The model under review builds one solid part; all positions refer to its coordinate system, in mm. Face numbers are marked on the shaded views. Give positions to 0.01 mm unless a question says otherwise; leave off trailing zeros. Loops run counter-clockwise (first coordinate to the right, second up) from the corner with the lowest first, then second, coordinate; pieces in that order, holes last. Notation, with made-up numbers: (9, 2) - (56, 2) arc R23 ccw to (56, 37) - close; hole circle Ø7 at (44, -21.75). An arc over 180 degrees is marked (long way). Return JSON: item names as keys, results as strings. Group by question number.
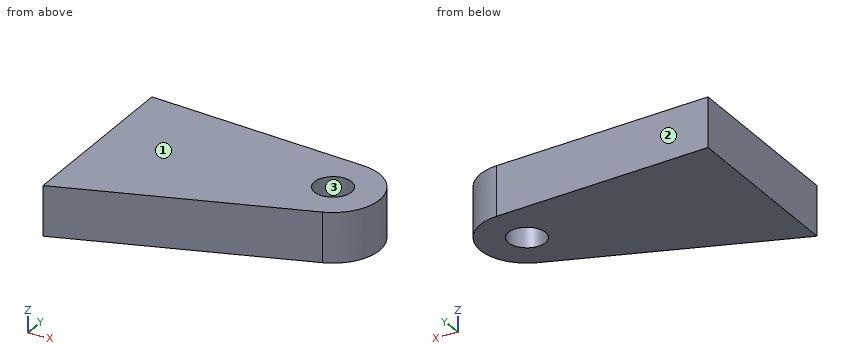
Autodesk Inventor part; units mm, degrees
ref_plane "YZ Plane" through (0, 0, 0) normal (1, 0, 0) x (0, 1, 0)
ref_plane "XZ Plane" through (0, 0, 0) normal (0, 1, 0) x (-1, 0, 0)
ref_plane "XY Plane" through (0, 0, 0) normal (0, 0, 1) x (1, 0, 0)
sketch "Sketch1" plane through (0, 0, 0) normal (0, 0, 1) x (1, 0, 0)
  circle A0 centre (0, 0) radius 3
  arc A1 (2.4445, -7.0904) -> (0.5304, 7.4812) centre (0, 0) ccw
  line L0 (-35, 10) -> (-35, -20)
  line L1 (-35, 10) -> (0.5304, 7.4812)
  line L2 (-35, -20) -> (2.4445, -7.0904)
  dimension "d0" = 6
  dimension "d1" = 15
  dimension "d2" = 35
  dimension "d3" = 10
  dimension "d4" = 30
extrude "Extrusion1" add sketch "Sketch1" against normal blind 8
properties part number "BaseHinge"
1) For pin 1 Ø4 at (y, z) = (6.5, -5) entering from +X; pin 2 Ø1 at (x, z) = (-5, -6.5) entering from -Y; pin 3 Ø2 at (x, y) = (-28, -11.5) entering from +Z; pin 4 Ø1.5 at (y, z) = (4.5, -7) entering from +X, all flat-tipped, find the tip position at first contact; note any pin that passes through.
2) We need section B-B, the plane x = 0. Write out the cut boundary in (y, z), plus the area to 3 significant figures.
3) We need section D-D, the plane y = -5.5. Write out the cut boundary in (x, z), plus the area to 3 significant figures.
4) We need section C-C, the plane z = -2.25. Write out the cut boundary in (x, y).
5) To check wall thickness, follow line 1 (Y direction, x = 0, z = -2); line 2 (X direction, y = -1.5, z = -0.5); line 3 (X direction, y = 5, z = -0.25). State the ranges of each line that lie inside material, in increasing order.
6) We need section A-A, the plane y = 0. Write out the cut boundary in (x, z).
7) Draft analysis for pull direction Y (two halves, no side actions). For the marked faces 1, 2 and 3, state which applies: +Y half, -Y half, draft (parallel to the pull), parting line (faces both ways), or undercut.
Findings:
{
 "1": {"pin 1": "stops at x = 6", "pin 2": "stops at y = -9.83", "pin 3": "stops at z = 0", "pin 4": "stops at x = 6.5"},
 "2": {"outline": "(-7.93, -8) - (-3, -8) - (-3, 0) - (-7.93, 0) - close; (3, -8) - (7.52, -8) - (7.52, 0) - (3, 0) - close", "area": "75.6 mm^2"},
 "3": {"outline": "(-35, -8) - (5.1, -8) - (5.1, 0) - (-35, 0) - close", "area": "321 mm^2"},
 "4": {"outline": "(-35, -20) - (2.44, -7.09) arc R7.5 ccw to (0.53, 7.48) - (-35, 10) - close; hole circle Ø6 at (0, 0)"},
 "5": {"line 1": "y = -7.93 to -3, 3 to 7.52", "line 2": "x = -35 to -2.6, 2.6 to 7.35", "line 3": "x = -35 to 5.59"},
 "6": {"outline": "(-35, -8) - (-3, -8) - (-3, 0) - (-35, 0) - close; (3, -8) - (7.5, -8) - (7.5, 0) - (3, 0) - close"},
 "7": {"face 1": "draft", "face 2": "+Y half", "face 3": "undercut"}
}
